Part model, mm, in its own coordinate system. Face numbers are marked on the shaded views. A direction names the side the tool comes from. Coordinates: 2 decimals unless noted, no trailing zeros. Loops run counter-clockwise (first coordinate to the right, second up) from the corner with the lowest first, then second, coordinate; pieces in that order, holes last. Notation, with made-up numbers: (24.25, 48.25) -> (46.25, 48.25) arc R15 ccw to (46.25, 55.25) -> close; hole circle Ø4 at (-35.75, -39.75). An arc over 180 degrees is marked (long way). One line per item, written item: value. Start each with the question number.
from build123d import *

# Parameters (mm, degrees)
EXTRUDE_1_DEPTH     = 4
SKETCH_2_W          = 4
SKETCH_2_H          = 5
EXTRUDE_2_DEPTH     = 6
SKETCH_3_R          = 0.95
CUT_EXTRUDE_1_DEPTH = 53.607604013
SKETCH_4_R          = 1
CUT_EXTRUDE_2_DEPTH = 52.995769059


with BuildPart() as part:
    # 草图1 → 凸台-拉伸1 (new body)
    with BuildSketch(Plane(origin=(0, 0, 0), x_dir=(1, 0, 0), z_dir=(0, 1, 0))):
        Polygon((0, 0), (0, -5), (20, -5), (23.4, -5), (43.4, -5), (43.4, 0), (27.4, 0), (27.4, 23), (43.4, 23), (43.4, 28), (23.4, 28), (20, 28), (0, 28), (0, 23), (16, 23), (16, 0), align=None)
    extrude(amount=EXTRUDE_1_DEPTH)

    # 草图2 → 凸台-拉伸2 (add)
    with BuildSketch(Plane(origin=(0, 4, 0), x_dir=(1, 0, 0), z_dir=(0, 1, 0))):
        with Locations((2, -2.5)):
            Rectangle(SKETCH_2_W, SKETCH_2_H)
        with Locations((2, 25.5)):
            Rectangle(SKETCH_2_W, SKETCH_2_H)
        with Locations((41.4, -2.5)):
            Rectangle(SKETCH_2_W, SKETCH_2_H)
        with Locations((41.4, 25.5)):
            Rectangle(SKETCH_2_W, SKETCH_2_H)
    extrude(amount=EXTRUDE_2_DEPTH)

    # 草图3 → 切除-拉伸1 (cut, through all)
    with BuildSketch(Plane.ZY):
        with Locations((2.5, 6)):
            Circle(SKETCH_3_R)
        with Locations((-25.5, 6)):
            Circle(SKETCH_3_R)
    extrude(amount=-CUT_EXTRUDE_1_DEPTH, mode=Mode.SUBTRACT)

    # 草图4 → 切除-拉伸2 (cut, through all)
    with BuildSketch(Plane(origin=(0, 4, 0), x_dir=(1, 0, 0), z_dir=(0, 1, 0))):
        with Locations(Location((7, -2.5, 0), (0, 0, 270))):
            Circle(SKETCH_4_R)
        with Locations(Location((7, 25.5, 0), (0, 0, 270))):
            Circle(SKETCH_4_R)
        with Locations(Location((18, 11.5, 0), (0, 0, 270))):
            Circle(SKETCH_4_R)
        with Locations(Location((36.4, -2.5, 0), (0, 0, 90))):
            Circle(SKETCH_4_R)
        with Locations(Location((36.4, 25.5, 0), (0, 0, 90))):
            Circle(SKETCH_4_R)
        with Locations(Location((25.4, 11.5, 0), (0, 0, 90))):
            Circle(SKETCH_4_R)
    extrude(amount=-CUT_EXTRUDE_2_DEPTH, mode=Mode.SUBTRACT)


solid = part.part
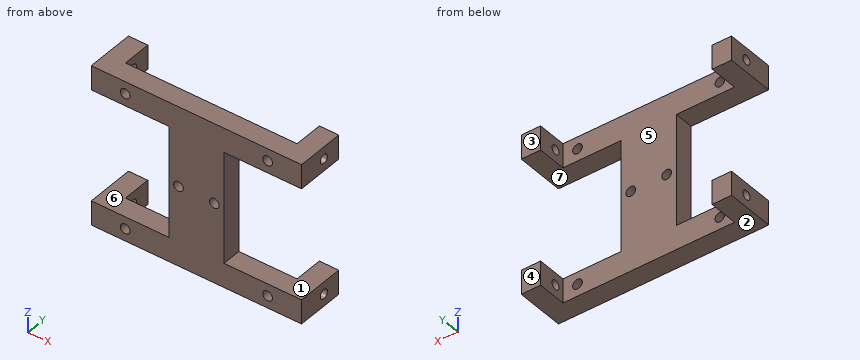
1) Slice it at C-C (y = 0.75). Give the cut face in (x, z), then the cut area to 3 significant figures.
2) Slice it at A-A (z = -11.5). Give the cut face in (x, y), then the cut area to 3 significant figures.
3) Probe line 1 (X direction, y = 3.1, z = -11.5); line 2 (X direction, y = 0.9, z = -25.5); line 3 (Z direction, x = 36.4, y = 1.65). List the from-to ranges inside material, lowest first. Write a range as from..to.
4) Slice it at B-B (z = -25.5). Give the cut face in (x, y).
5) Pull direction Z, two halves, no side cores. Call the marked faces 1, 2 and 3: +Z half, -Z half, draft (parallel to the pull), parting line (faces both ways), or undercut.
6) Slice it at D-D (x = 36.4). Give the cut face in (y, z).
7) Pin check, flat tips, straight feed: pin 1 Ø1.7 at (y, z) = (6, 2.5) entering from -X; pin 2 Ø2 at (y, z) = (3.5, -11) entering from -X; pin 3 Ø3 at (x, z) = (7, -25.5) entering from +Y. Stop position of each tip, or through.
8) Tool access for the marked faces 4, 5, 6 and 7: list every direction of +Z, -Z, +X, -X, +Y, -Y with a clear straight run to the whole face (end or side of a thin tool).
Check sheet entries:
1. outline: (0, -28) -> (43.4, -28) -> (43.4, -23) -> (27.4, -23) -> (27.4, 0) -> (43.4, 0) -> (43.4, 5) -> (0, 5) -> (0, 0) -> (16, 0) -> (16, -23) -> (0, -23) -> close; hole circle Ø2 at (7, -25.5); hole circle Ø2 at (7, 2.5); hole circle Ø2 at (18, -11.5); hole circle Ø2 at (25.4, -11.5); hole circle Ø2 at (36.4, -25.5); hole circle Ø2 at (36.4, 2.5)
1. area: 677 mm^2
2. outline: (16, 0) -> (17, 0) -> (17, 4) -> (16, 4) -> close; (19, 0) -> (24.4, 0) -> (24.4, 4) -> (19, 4) -> close; (26.4, 0) -> (27.4, 0) -> (27.4, 4) -> (26.4, 4) -> close
2. area: 29.6 mm^2
3. line 1: x = 16..17, 19..24.4, 26.4..27.4
3. line 2: x = 0..6, 8..35.4, 37.4..43.4
3. line 3: z = -28..-26.5, -24.5..-23, 0..1.5, 3.5..5
4. outline: (0, 0) -> (6, 0) -> (6, 4) -> (4, 4) -> (4, 5.05) -> (0, 5.05) -> close; (0, 6.95) -> (4, 6.95) -> (4, 10) -> (0, 10) -> close; (8, 0) -> (35.4, 0) -> (35.4, 4) -> (8, 4) -> close; (37.4, 0) -> (43.4, 0) -> (43.4, 5.05) -> (39.4, 5.05) -> (39.4, 4) -> (37.4, 4) -> close; (39.4, 6.95) -> (43.4, 6.95) -> (43.4, 10) -> (39.4, 10) -> close
5. face 1: undercut
5. face 2: -Z half
5. face 3: draft
6. outline: (0, -28) -> (4, -28) -> (4, -26.5) -> (0, -26.5) -> close; (0, -24.5) -> (4, -24.5) -> (4, -23) -> (0, -23) -> close; (0, 0) -> (4, 0) -> (4, 1.5) -> (0, 1.5) -> close; (0, 3.5) -> (4, 3.5) -> (4, 5) -> (0, 5) -> close
7. pin 1: passes through
7. pin 2: stops at x = 16
7. pin 3: stops at y = 4
8. face 4: +Z, -Z, +X, -X, +Y
8. face 5: +Z, -Z, +Y
8. face 6: -X, +Y, -Y
8. face 7: +X, +Y, -Y
